```python
from build123d import *

# Parameters (mm, degrees)
F1_DEPTH = 62
F2_R     = 2
F3_DEPTH = 29.301
F4_W     = 48
F4_H     = 7
F5_DEPTH = 29.301
F6_R     = 1
F7_R     = 5
F8_W     = 29.3
F8_H     = 7
F9_DEPTH = 1.5
F10_R    = 1


with BuildPart() as f1:
    # F0 (on Front) → F1 (new body)
    with BuildSketch(Plane.XZ):
        Polygon((0, 11.5), (0, 0), (1.5, 0), (1.5, 10), (27.8, 10), (27.8, 0), (29.3, 0), (29.3, 11.5), align=None)
    extrude(amount=F1_DEPTH)

    # F2 (on face) → F3 (cut, through all)
    with BuildSketch(Plane.YZ.offset(29.3)):
        with Locations((-58.5, 6.5)):
            Circle(F2_R)
        with Locations((-3.5, 6.5)):
            Circle(F2_R)
    extrude(amount=-F3_DEPTH, mode=Mode.SUBTRACT)

    # F4 (on face) → F5 (cut, through all)
    with BuildSketch(Plane.YZ.offset(29.3)):
        with Locations((-31, 3.5)):
            Rectangle(F4_W, F4_H)
    extrude(amount=-F5_DEPTH, mode=Mode.SUBTRACT)

    # F6
    f6_edges = [f1.edges().sort_by_distance(p)[0] for p in [
        (28.55, -62, 0),
        (0.75, -55, 0),
        (28.55, -55, 0),
        (0.75, -62, 0),
        (28.55, 0, 0),
        (0.75, -7, 0),
        (28.55, -7, 0),
        (0.75, 0, 0),
    ]]
    fillet(f6_edges, radius=F6_R)

    # F7
    f7_edges = [f1.edges().sort_by_distance(p)[0] for p in [
        (0.75, -7, 7),
        (28.55, -7, 7),
        (0.75, -55, 7),
        (28.55, -55, 7),
    ]]
    fillet(f7_edges, radius=F7_R)

    # F8 (on face) → F9 (cut)
    with BuildSketch(Plane.XY.offset(11.5)):
        with Locations((14.65, -58.5)):
            Rectangle(F8_W, F8_H)
        with Locations((14.65, -3.5)):
            Rectangle(F8_W, F8_H)
    extrude(amount=-F9_DEPTH, mode=Mode.SUBTRACT)

    # F10
    f10_edges = [f1.edges().sort_by_distance(p)[0] for p in [
        (0.75, -62, 10),
        (28.55, -62, 10),
        (0.75, 0, 10),
        (28.55, 0, 10),
    ]]
    fillet(f10_edges, radius=F10_R)


solid = f1.part
```
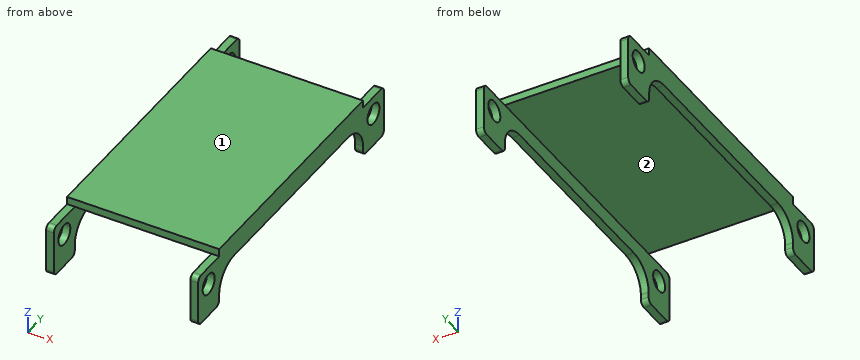
For this review, take the finished solid that the model builds, in its own axes (mm). Face numbers are marked on the shaded views. A direction names the side the tool comes from. Coordinates: 2 decimals unless noted, no trailing zeros. Write each loop counter-clockwise with the first axis right and the second up, starting at its lowest first coordinate (ties: lowest second). Pieces come first, ordered by that corner, then holes. Notation, with made-up numbers: (89, 44.25) - (103, 44.25) arc R17 cw to (103, 52.25) - close; hole circle Ø11 at (77.5, 89.25). An arc over 180 degrees is marked (long way). Put each result on its own line as item: value.
1. Machinability: for the marked faces 1 and 2, which of the approach directions +Z, -Z, +X, -X, +Y, -Y give a long, thin tool a straight path to every point of the face, cutting with its end or side? Answer none if there is none.
Values found:
face 1: +Z, +X, -X, +Y, -Y
face 2: -Z, +Y, -Y
2. Add section C-C, the plane y = -46.5. Give the boundary of the cut face in (x, z).
Values found:
outline: (0, 7) - (1.5, 7) - (1.5, 10) - (27.8, 10) - (27.8, 7) - (29.3, 7) - (29.3, 11.5) - (0, 11.5) - close
3. Add section D-D, the plane x = 9. Give the boundary of the cut face in (y, z), then the cut area to 3 significant figures.
Values found:
outline: (-55, 10) - (-7, 10) - (-7, 11.5) - (-55, 11.5) - close
area: 72.0 mm²
4. Add section B-B, the plane z = 5.75. Count the separate pieces of the cut face and the enclosed holes in it, then the cut area to 3 significant figures.
Values found:
separate pieces: 8
enclosed holes: 0
area: 29.9 mm²
5. Add section A-A, the plane y = -3.5. Give the boundary of the cut face in (x, z).
Values found:
outline: (0, 0) - (1.5, 0) - (1.5, 4.5) - (0, 4.5) - close; (0, 8.5) - (1.5, 8.5) - (1.5, 10) - (0, 10) - close; (27.8, 0) - (29.3, 0) - (29.3, 4.5) - (27.8, 4.5) - close; (27.8, 8.5) - (29.3, 8.5) - (29.3, 10) - (27.8, 10) - close
6. For pin 1 (8 mm diameter, centred on x = 24.5, y = -45.5, fed in from -Z); pin 2 (10 mm diameter, centred on x = 21, y = -50.5, fed in from -Z); pin 3 (1.2 mm diameter, centred on x = 28.5, y = -58, fed in from +Z); pin 4 (1 mm diameter, centred on x = 16, z = 9, fed in from +Y), all flat-tipped, find the tip position at first contact; note any pin that passes through.
Values found:
pin 1: z = 7
pin 2: z = 10
pin 3: z = 10
pin 4: through
7. Wall thickness on probe 1 along Z at (x, y) = (28.85, -3.5); probe 2 along X at (y, z) = (-24, 8.75); probe 3 along Z at (x, y) = (10.25, -40.5): over which ranges is each line inside the solid? List them lowest first.
Values found:
probe 1: 0 to 4.5, 8.5 to 10
probe 2: 0 to 1.5, 27.8 to 29.3
probe 3: 10 to 11.5
